```python
from build123d import *

# Parameters (mm, degrees)
BOSS_EXTRUDE1_DEPTH = 75
CUT_EXTRUDE2_REACH  = 202.429
SKETCH4_R           = 2.05
SKETCH4_3_R         = 3.5
SKETCH4_3_R_2       = 2.05
CUT_EXTRUDE3_DEPTH  = 4
SKETCH5_W           = 70.551930768
SKETCH5_H           = 5
BOSS_EXTRUDE2_DEPTH = 2
SKETCH6_R           = 2.15
CUT_EXTRUDE4_DEPTH  = 5
FILLET1_R           = 1


with BuildPart() as part:
    # Sketch2 → Boss-Extrude1 (new body)
    with BuildSketch(Plane.XY):
        with BuildLine():
            Line((-88.5, -160.346147872), (-88.5, -7))
            Line((-88.5, -7), (-26, -7))
            Line((-26, -7), (-26, 0))
            Line((-26, 0), (-93, 0))
            ThreePointArc((-93, 0), (-93.707106781, -0.292893219), (-94, -1))
            Line((-94, -1), (-94, -160.346147872))
            Line((-94, -160.346147872), (-88.5, -160.346147872))
        make_face()
    extrude(amount=BOSS_EXTRUDE1_DEPTH)

    # Sketch4 → Cut-Extrude2 (cut, up to next)
    with BuildSketch(Plane(origin=(0, 0, 0), x_dir=(1, 0, 0), z_dir=(0, 1, 0)), mode=Mode.PRIVATE) as cut_extrude2_sk1:
        with Locations(Location((-30.341713377, -5, 0), (0, 0, 270))):
            Circle(SKETCH4_R)
    cut_extrude2_tool1 = extrude(cut_extrude2_sk1.sketch, amount=-CUT_EXTRUDE2_REACH, mode=Mode.PRIVATE) & part.part
    # Sketch4 → Cut-Extrude2 (cut, up to next)
    with BuildSketch(Plane(origin=(0, 0, 0), x_dir=(1, 0, 0), z_dir=(0, 1, 0)), mode=Mode.PRIVATE) as cut_extrude2_sk2:
        with Locations(Location((-30.341713377, -70, 0), (0, 0, 270))):
            Circle(SKETCH4_R)
    cut_extrude2_tool2 = extrude(cut_extrude2_sk2.sketch, amount=-CUT_EXTRUDE2_REACH, mode=Mode.PRIVATE) & part.part
    add(cut_extrude2_tool1.solids().sort_by_distance((-30.341713, 0, 5))[0], mode=Mode.SUBTRACT)
    add(cut_extrude2_tool2.solids().sort_by_distance((-30.341713, 0, 70))[0], mode=Mode.SUBTRACT)

    # Sketch4<3> → Cut-Extrude3 (cut)
    # profile 1 of 2: a face of its own
    with BuildSketch(Plane(origin=(0, 0, 0), x_dir=(1, 0, 0), z_dir=(0, 1, 0))):
        with Locations(Location((-30.341713377, -5, 0), (0, 0, 270))):
            Circle(SKETCH4_3_R)
        with Locations(Location((-30.341713377, -5, 0), (0, 0, 270))):
            Circle(SKETCH4_3_R_2, mode=Mode.SUBTRACT)
    # profile 2 of 2: a face of its own
    with BuildSketch(Plane(origin=(0, 0, 0), x_dir=(1, 0, 0), z_dir=(0, 1, 0))):
        with Locations(Location((-30.341713377, -70, 0), (0, 0, 270))):
            Circle(SKETCH4_3_R)
        with Locations(Location((-30.341713377, -70, 0), (0, 0, 270))):
            Circle(SKETCH4_3_R_2, mode=Mode.SUBTRACT)
    extrude(amount=-CUT_EXTRUDE3_DEPTH, mode=Mode.SUBTRACT)

    # Sketch5 → Boss-Extrude2 (add)
    with BuildSketch(Plane(origin=(-88.5, 0, 0), x_dir=(0, 0, -1), z_dir=(1, 0, 0))):
        with Locations((-39.724034616, -157.846147872)):
            Rectangle(SKETCH5_W, SKETCH5_H)
    extrude(amount=BOSS_EXTRUDE2_DEPTH)

    # Sketch6 → Cut-Extrude4 (cut)
    with BuildSketch(Plane.XZ.offset(160.346147872)):
        with Locations(Location((-89.75, 10, 0), (0, 0, 270))):
            Circle(SKETCH6_R)
        with Locations(Location((-89.75, 65, 0), (0, 0, 270))):
            Circle(SKETCH6_R)
    extrude(amount=-CUT_EXTRUDE4_DEPTH, mode=Mode.SUBTRACT)

    # Fillet1
    fillet1_edges = [part.edges().sort_by_distance(p)[0] for p in [
        (-94, -80.673073936, 75),
        (-93.707106781, -0.292893219, 75),
        (-59.5, 0, 75),
    ]]
    fillet(fillet1_edges, radius=FILLET1_R)


solid = part.part
```
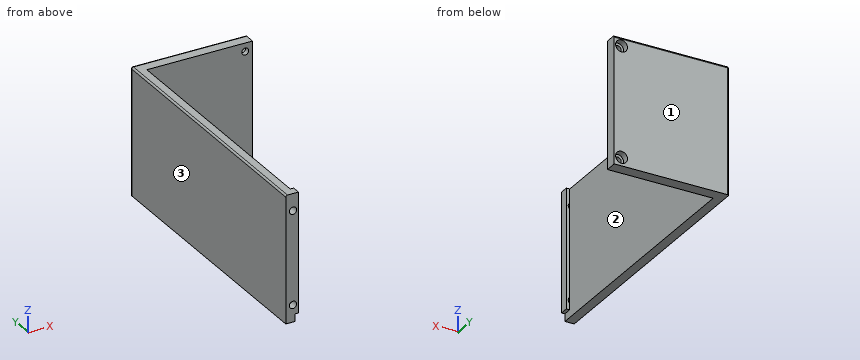
CAD build for the part. Positions are in the model's coordinates, mm. Face numbers are marked on the shaded views. Round coordinates to 2 decimals unless told otherwise and drop trailing zeros. Order: outer loops, then holes, each group sorted by start corner. A loop starts at its lowest first (then second) coordinate and runs counter-clockwise, first axis right, second up. Notation, with made-up numbers: (16.5, -24.75) - (27.5, -24.75) arc R11 cw to (27.5, -7.75) - close; hole circle Ø3 at (43.25, 55). An arc over 180 degrees is marked (long way). Answer in a Markdown table with one row per item. Add a question column.
(1) Band-saw the part on B-B on z = 54. List the corners of the cut face in (x, y), and give its area (3 significant figures).
(2) Band-saw the part on C-C on x = -54. List the corners of the cut face in (y, z).
(3) Mould opens along Y. For the marked faces 1, 2 and 3 say: +Y half, -Y half, draft (parallel to the pull), parting line (faces both ways), or undercut.
(4) Drop flat-ended pins along their axis: pin 1 Ø2 at (y, z) = (-43, 66) entering from +X; pin 2 Ø4.5 at (x, z) = (-30.34, 5) entering from +Y; pin 3 Ø1 at (x, z) = (-91, 64.5) entering from -Y. Give the stop position or say it passes through.
(5) Band-saw the part on A-A on z = 70. List the corners of the cut face in (x, y), and give its area (3 significant figures).
(6) Probe L1, parallel to X at y = -6.3, z = 5; L2, parallel to X at y = -159.1, z = 10; L3, parallel to Z at x = -89, y = -158. List the from-to ranges inside material, lowest first. Write a range as [from, to].
(7) Band-saw the part on D-D on y = -28. List the corners of the cut face in (x, z), and give its area (3 significant figures).
Data:
| question | item | result |
|---|---|---|
| 1 | outline | (-94, -160.35) - (-86.5, -160.35) - (-86.5, -155.35) - (-88.5, -155.35) - (-88.5, -7) - (-26, -7) - (-26, 0) - (-93, 0) arc R1 ccw to (-94, -1) - close |
| 1 | area | 1,330 mm^2 |
| 2 | outline | (-7, 0) - (0, 0) - (0, 74) arc R1 ccw to (-1, 75) - (-7, 75) - close |
| 3 | face 1 | +Y half |
| 3 | face 2 | undercut |
| 3 | face 3 | draft |
| 4 | pin 1 | stops at x = -88.5 |
| 4 | pin 2 | stops at y = -4 |
| 4 | pin 3 | stops at y = -155.35 |
| 5 | outline | (-94, -160.35) - (-86.5, -160.35) - (-86.5, -155.35) - (-88.5, -155.35) - (-88.5, -7) - (-32.39, -7) - (-32.39, -4) - (-33.84, -4) - (-33.84, 0) - (-93, 0) arc R1 ccw to (-94, -1) - close; (-28.29, -7) - (-26, -7) - (-26, 0) - (-26.84, 0) - (-26.84, -4) - (-28.29, -4) - close |
| 5 | area | 1,290 mm^2 |
| 6 | L1 | x = [-94, -32.39], [-28.29, -26] |
| 6 | L2 | x = [-94, -91.9], [-87.6, -86.5] |
| 6 | L3 | z = [0, 7.99], [12.01, 62.99], [67.01, 75] |
| 7 | outline | (-94, 0) - (-88.5, 0) - (-88.5, 75) - (-93, 75) arc R1 ccw to (-94, 74) - close |
| 7 | area | 412 mm^2 |
